Input: dimensioned drawing with shaded views. Units: mm. Origin: part minimum x, y, z. Round coordinates to 2 decimals unless told otherwise and drop trailing zeros. Write each loop counter-clockwise with the first axis right and the second up, starting at its lowest first coordinate (ties: lowest second). Pieces come first, ordered by that corner, then holes. Notation, with made-up numbers: (-14, -16) - (28, -16) arc R15 ccw to (28, -7) - close; hole circle Ø11 at (41.25, 22). An arc over 180 degrees is marked (long way). Use one line per item in the form item = value.
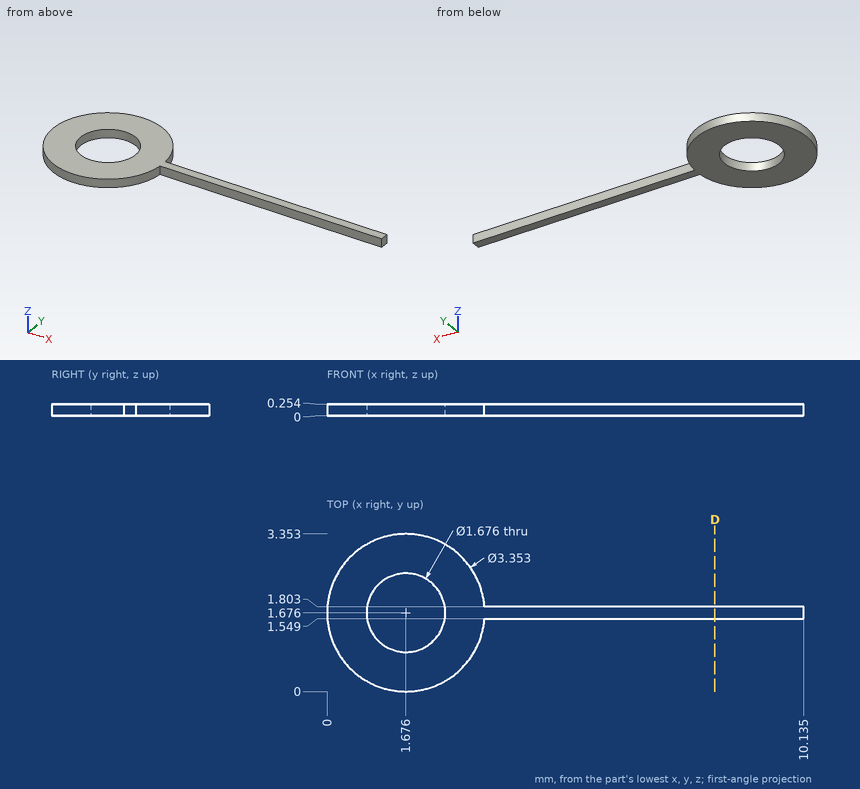
(1) Material intervals for L1, parallel to Y at x = 7.25, z = 0.1; L2, parallel to X at y = 2.35, z = 0.2 (1 decimal); L3, parallel to X at y = 1.45, z = 0.1 (1 decimal), sorted ascending.
Derived:
L1 = 1.55 to 1.8
L2 = 0.1 to 1.2, 2.2 to 3.2
L3 = 0 to 0.9, 2.5 to 3.3
(2) First-contact query: pin 1 Ø2 at (x, y) = (1.68, 1.68) entering from -Z. Flat tip, straight axial feed; report the tip coordinate or a pass-through.
Derived:
pin_1 = 0
(3) Cut plane D-D on x = 8.25. Output: boundary loops of the cut face in (y, z).
Derived:
outline = (1.55, 0) - (1.8, 0) - (1.8, 0.25) - (1.55, 0.25) - close
